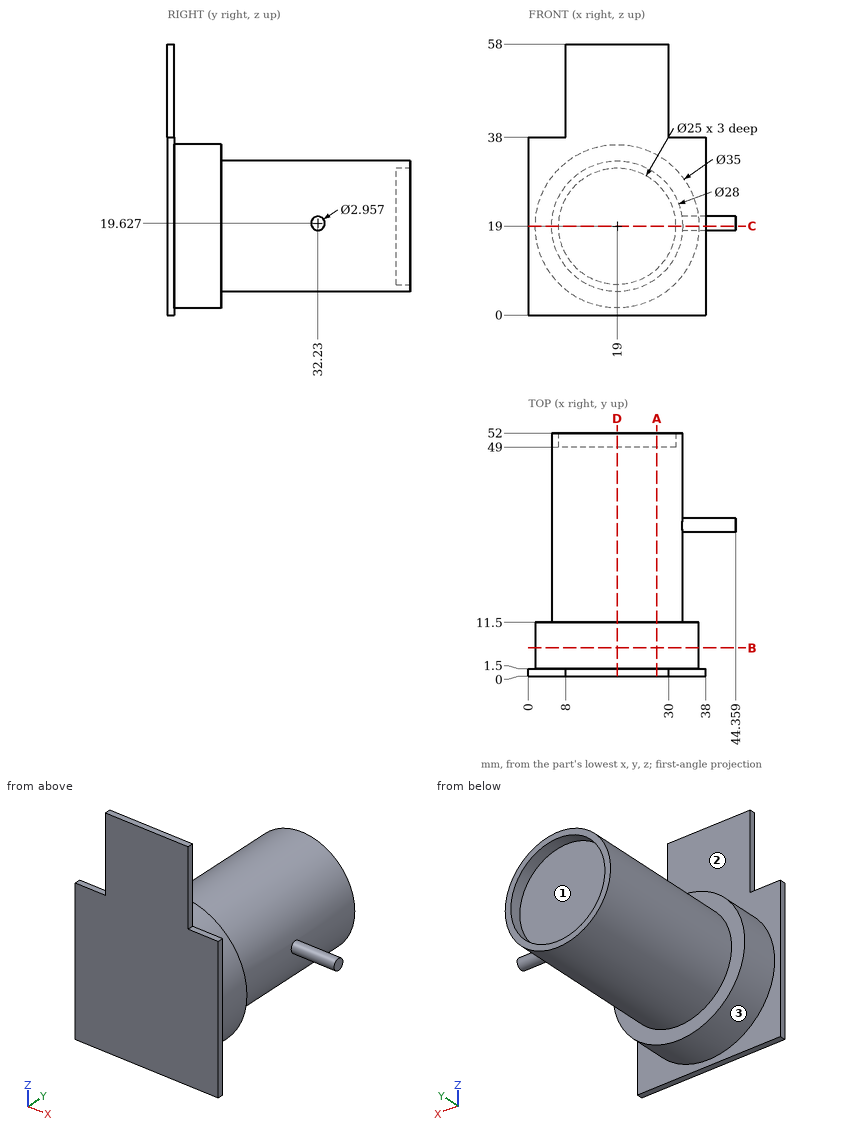
Input: dimensioned drawing with shaded views. Units: mm. Origin: part minimum x, y, z. Round coordinates to 2 decimals unless told otherwise and drop trailing zeros. Loops run counter-clockwise (first coordinate to the right, second up) from the corner with the lowest first, then second, coordinate; pieces in that order, holes last. Notation, with made-up numbers: (-30.5, -29) -> (-9.5, -29) arc R27 cw to (-9.5, -6) -> close; hole circle Ø11 at (-5.75, 82). An arc over 180 degrees is marked (long way). Use one line per item in the form item = value. Start each with the question number.
1) Section A-A on x = 27.5. Output: boundary loops of the cut face in (y, z) (1 decimal).
2) Section D-D on x = 19. Output: boundary loops of the cut face in (y, z), then the cut area to 3 significant figures.
3) Section B-B on y = 6. Output: boundary loops of the cut face in (x, z), then the cut area to 3 significant figures.
4) Draft query along X for the marked faces 1, 2 and 3. Return one class per face: released by +X, released by -X, zero draft, split by the parting line, or undercut.
5) Section C-C on z = 19. Output: boundary loops of the cut face in (x, y).
6) Line query: L1, parallel to X at y = 50, z = 19; L2, parallel to Y at x = 20, z = 21. Output: solid intervals per line, ascending.
7) First-contact query: P1, Ø7.5, axis at x = 14, z = 22, coming from the +Y side; P2, Ø1.6, axis at y = 0.5, z = 52, coming from the -X side; P3, Ø1.6, axis at x = 6, y = 0.5, coming from the +Z side. Flat tips, straight axial feed; report the tip coordinate or a pass-through.
Response:
q1.outline = (0, 0) -> (1.5, 0) -> (1.5, 3.7) -> (11.5, 3.7) -> (11.5, 7.9) -> (52, 7.9) -> (52, 9.8) -> (49, 9.8) -> (49, 28.2) -> (52, 28.2) -> (52, 30.1) -> (11.5, 30.1) -> (11.5, 34.3) -> (1.5, 34.3) -> (1.5, 58) -> (0, 58) -> close
q2.outline = (0, 0) -> (1.5, 0) -> (1.5, 1.5) -> (11.5, 1.5) -> (11.5, 5) -> (52, 5) -> (52, 6.5) -> (49, 6.5) -> (49, 31.5) -> (52, 31.5) -> (52, 33) -> (11.5, 33) -> (11.5, 36.5) -> (1.5, 36.5) -> (1.5, 58) -> (0, 58) -> close
q2.area = 1,500 mm^2
q3.outline = circle Ø35 at (19, 19)
q3.area = 962 mm^2
q4.face_1 = undercut
q4.face_2 = zero draft
q4.face_3 = split by the parting line
q5.outline = (0, 0) -> (38, 0) -> (38, 1.5) -> (36.5, 1.5) -> (36.5, 11.5) -> (33, 11.5) -> (33, 30.89) -> (44.36, 30.89) -> (44.36, 33.57) -> (33, 33.57) -> (33, 52) -> (31.5, 52) -> (31.5, 49) -> (6.5, 49) -> (6.5, 52) -> (5, 52) -> (5, 11.5) -> (1.5, 11.5) -> (1.5, 1.5) -> (0, 1.5) -> close
q6.L1 = 5 to 6.5, 31.5 to 33
q6.L2 = 0 to 49
q7.P1 = 49
q7.P2 = 8
q7.P3 = 38
